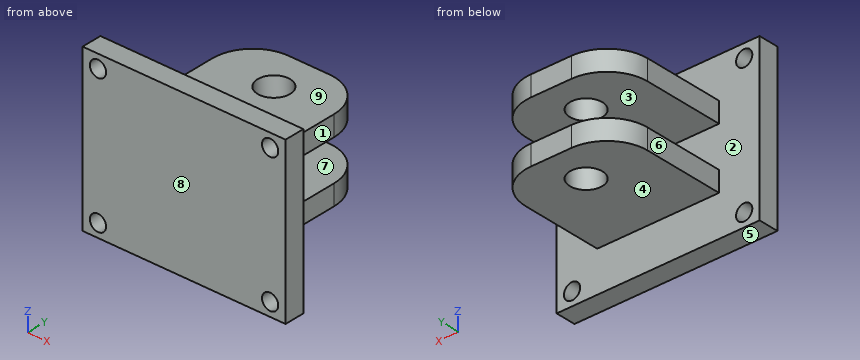
from build123d import *

# Parameters (mm, degrees)
SKETCH1_W           = 50
SKETCH1_H           = 40
BOSS_EXTRUDE1_DEPTH = 5
SKETCH2_W           = 30
SKETCH2_H           = 5
BOSS_EXTRUDE2_DEPTH = 35
FILLET1_R           = 10
FILLET2_R           = 10
FILLET3_R           = 10
FILLET4_R           = 10
SKETCH3_R           = 4
CUT_EXTRUDE1_DEPTH  = 35
SKETCH5_R           = 2
CUT_EXTRUDE3_DEPTH  = 35
SKETCH5_4_R         = 2
CUT_EXTRUDE4_DEPTH  = 35


with BuildPart() as part:
    # Sketch1 → Boss-Extrude1 (new body)
    with BuildSketch(Plane(origin=(0, 0, 0), x_dir=(1, 0, 0), z_dir=(0, 1, 0))):
        with Locations((2.66798419, -7.845849802)):
            Rectangle(SKETCH1_W, SKETCH1_H)
    extrude(amount=BOSS_EXTRUDE1_DEPTH)

    # Sketch2 → Boss-Extrude2 (add)
    with BuildSketch(Plane(origin=(0, 0, 0), x_dir=(1, 0, 0), z_dir=(0, 1, 0))):
        with Locations((2.66798419, -15.345849802)):
            Rectangle(SKETCH2_W, SKETCH2_H)
        with Locations((2.66798419, -0.345849802)):
            Rectangle(SKETCH2_W, SKETCH2_H)
    extrude(amount=BOSS_EXTRUDE2_DEPTH)

    # Fillet1
    fillet1_edges = [part.edges().sort_by_distance(p)[0] for p in [
        (17.66798419, 35, 15.345849802),
    ]]
    fillet(fillet1_edges, radius=FILLET1_R)

    # Fillet2
    fillet2_edges = [part.edges().sort_by_distance(p)[0] for p in [
        (-12.33201581, 35, 15.345849802),
    ]]
    fillet(fillet2_edges, radius=FILLET2_R)

    # Fillet3
    fillet3_edges = [part.edges().sort_by_distance(p)[0] for p in [
        (-12.33201581, 35, 0.345849802),
    ]]
    fillet(fillet3_edges, radius=FILLET3_R)

    # Fillet4
    fillet4_edges = [part.edges().sort_by_distance(p)[0] for p in [
        (17.66798419, 35, 0.345849802),
    ]]
    fillet(fillet4_edges, radius=FILLET4_R)

    # Sketch3 → Cut-Extrude1 (cut)
    with BuildSketch(Plane.XY.offset(17.845849802)):
        with Locations((2.834176639, 25)):
            Circle(SKETCH3_R)
    extrude(amount=-CUT_EXTRUDE1_DEPTH, mode=Mode.SUBTRACT)

    # Sketch5 → Cut-Extrude3 (cut)
    with BuildSketch(Plane(origin=(0, 5, 0), x_dir=(1, 0, 0), z_dir=(0, 1, 0))):
        with Locations(Location((-18.537983824, 8.872799407, 0), (0, 0, 270))):
            Circle(SKETCH5_R)
    extrude(amount=-CUT_EXTRUDE3_DEPTH, mode=Mode.SUBTRACT)

    # Sketch5<4> → Cut-Extrude4 (cut)
    with BuildSketch(Plane(origin=(0, 5, 0), x_dir=(1, 0, 0), z_dir=(0, 1, 0))):
        with Locations(Location((23.873952204, -24.564499012, 0), (0, 0, 270))):
            Circle(SKETCH5_4_R)
        with Locations(Location((-18.537983824, -24.564499012, 0), (0, 0, 270))):
            Circle(SKETCH5_4_R)
        with Locations(Location((23.873952204, 8.872799407, 0), (0, 0, 270))):
            Circle(SKETCH5_4_R)
        with Locations(Location((-18.537983824, 8.872799407, 0), (0, 0, 270))):
            Circle(SKETCH5_4_R)
    extrude(amount=-CUT_EXTRUDE4_DEPTH, mode=Mode.SUBTRACT)


solid = part.part
CAD build for the part. Positions are in the model's coordinates, mm. Face numbers are marked on the shaded views. A direction names the side the tool comes from. Give positions to 0.01 mm unless a question says otherwise; leave off trailing zeros. Write each loop counter-clockwise with the first axis right and the second up, starting at its lowest first coordinate (ties: lowest second). Pieces come first, ordered by that corner, then holes. Notation, with made-up numbers: (-40, -18) -> (-2, -18) arc R22 cw to (-2, -1) -> close; hole circle Ø8 at (16, 40). An arc over 180 degrees is marked (long way). Return JSON: item names as keys, results as strings.
Item 1: Band-saw the part on B-B (x = 0.5). List the corners of the cut face in (y, z), then the cut area to 3 significant figures.
Answer below:
{"outline": "(0, -12.15) -> (5, -12.15) -> (5, -2.15) -> (21.75, -2.15) -> (21.75, 2.85) -> (5, 2.85) -> (5, 12.85) -> (21.75, 12.85) -> (21.75, 17.85) -> (5, 17.85) -> (5, 27.85) -> (0, 27.85) -> close; (28.25, -2.15) -> (35, -2.15) -> (35, 2.85) -> (28.25, 2.85) -> close; (28.25, 12.85) -> (35, 12.85) -> (35, 17.85) -> (28.25, 17.85) -> close", "area": "435 mm2"}
Item 2: Drop flat-ended pins along their axis: pin 1 (6 mm diameter, centred on x = -14, y = 15.5, fed in from +Z); pin 2 (1.5 mm diameter, centred on y = 14.5, z = 14.5, fed in from +X); pin 3 (2.5 mm diameter, centred on y = 10.5, z = 14, fed in from -X); pin 4 (3 mm diameter, centred on x = -18.54, z = 24.56, fed in from +Y). Give the stop position or say it passes through.
Answer below:
{"pin 1": "stops at z = 17.85", "pin 2": "stops at x = 17.67", "pin 3": "stops at x = -12.33", "pin 4": "passes through"}
Item 3: Tool access for the marked faces 5, 6, 7, 8 and 9: list every direction of +Z, -Z, +X, -X, +Y, -Y with a clear straight run to the whole face (end or side of a thin tool).
Answer below:
{"face 5": "-Z, +X, -X, +Y, -Y", "face 6": "+Z, -Z, -X, +Y", "face 7": "+X, -X, +Y", "face 8": "+Z, -Z, +X, -X, -Y", "face 9": "+Z, +X, -X, +Y"}
Item 4: Band-saw the part on A-A (y = 10.5). List the corners of the cut face in (x, z), then the cut area to 3 significant figures.
Answer below:
{"outline": "(-12.33, -2.15) -> (17.67, -2.15) -> (17.67, 2.85) -> (-12.33, 2.85) -> close; (-12.33, 12.85) -> (17.67, 12.85) -> (17.67, 17.85) -> (-12.33, 17.85) -> close", "area": "300 mm2"}
Item 5: Two-plate mould, pull along Z, no slides. Class the marked faces 1, 2, 3 and 4: +Z half, -Z half, draft (parallel to the pull), parting line (faces both ways), or undercut.
Answer below:
{"face 1": "draft", "face 2": "undercut", "face 3": "undercut", "face 4": "-Z half"}
Item 6: Drill centre lines: probe 1 along X at (y, z) = (3, 24.5) (3 decimals); probe 2 along Z at (x, y) = (-10, 7.5); probe 3 along X at (y, z) = (18, 17.5). Where is each one in solid material? Low to high.
Answer below:
{"probe 1": "x = -22.332 to -20.537, -16.539 to 21.875, 25.873 to 27.668", "probe 2": "z = -2.15 to 2.85, 12.85 to 17.85", "probe 3": "x = -12.33 to 17.67"}
Item 7: Band-saw the part on C-C (z = 16). List the corners of the cut face in (x, y).
Answer below:
{"outline": "(-22.33, 0) -> (27.67, 0) -> (27.67, 5) -> (17.67, 5) -> (17.67, 25) arc R10 ccw to (7.67, 35) -> (-2.33, 35) arc R10 ccw to (-12.33, 25) -> (-12.33, 5) -> (-22.33, 5) -> close; hole circle Ø8 at (2.83, 25)"}
Item 8: Band-saw the part on D-D (z = -9). List the corners of the cut face in (x, y), then the cut area to 3 significant figures.
Answer below:
{"outline": "(-22.33, 0) -> (-20.53, 0) -> (-20.53, 5) -> (-22.33, 5) -> close; (-16.54, 0) -> (21.88, 0) -> (21.88, 5) -> (-16.54, 5) -> close; (25.87, 0) -> (27.67, 0) -> (27.67, 5) -> (25.87, 5) -> close", "area": "210 mm2"}
